from build123d import *

# Parameters (mm, degrees)
CUT_EXTRUDE1_DEPTH = 2.5
FILLET1_R          = 0.5
CHAMFER1_SIZE      = 0.5


with BuildPart() as part:
    # Sketch1 → Revolve1 (revolve)
    with BuildSketch(Plane.XY, mode=Mode.PRIVATE) as revolve1_sk:
        Polygon((0, 0), (-6, 0), (-6, -0.5), (-3, -3.397066324), (-3, -12), (0, -12), align=None)
    revolve(revolve1_sk.sketch.rotate(Axis((0, 0, 0), (0, 1, 0)), 270), axis=Axis((0, 0, 0), (0, 1, 0)))

    # Sketch2 → Cut-Extrude1 (cut)
    with BuildSketch(Plane(origin=(0, 0, 0), x_dir=(1, 0, 0), z_dir=(0, 1, 0))):
        Polygon((0, 2.309401077), (-2, 1.154700538), (-2, -1.154700538), (0, -2.309401077), (2, -1.154700538), (2, 1.154700538), align=None)
    extrude(amount=-CUT_EXTRUDE1_DEPTH, mode=Mode.SUBTRACT)

    # Sketch3 → Cut-Revolve1 (revolve, cut)
    with BuildSketch(Plane.XY, mode=Mode.PRIVATE) as cut_revolve1_sk:
        Polygon((-2.31, 0), (-2, -0.260120886), (-2, -2.5), (0, -3.227940469), (0, 0), align=None)
    revolve(cut_revolve1_sk.sketch.rotate(Axis((0, -3.227940469, 0), (0, -1, 0)), 270), axis=Axis((0, -3.227940469, 0), (0, -1, 0)), mode=Mode.SUBTRACT)

    # Fillet1
    fillet1_edges = [part.edges().sort_by_distance(p)[0] for p in [
        (0, -3.397066324, 3),
    ]]
    fillet(fillet1_edges, radius=FILLET1_R)

    # Chamfer1
    chamfer1_edges = [part.edges().sort_by_distance(p)[0] for p in [
        (0, -12, 3),
    ]]
    chamfer(chamfer1_edges, length=CHAMFER1_SIZE)


solid = part.part
Input: part model. Units: mm. Frame: model coordinates. A direction names the side the tool comes from. Round coordinates to 2 decimals unless told otherwise and drop trailing zeros. Order: outer loops, then holes, each group sorted by start corner. A loop starts at its lowest first (then second) coordinate and runs counter-clockwise, first axis right, second up. Notation, with made-up numbers: (-11, 28.5) - (47, 28.5) arc R20 cw to (47, 44.5) - close; hole circle Ø6 at (-31.75, 8.5). An arc over 180 degrees is marked (long way). Answer as a JSON object with one key per item and string values. Group by question number.
(1) Cut plane B-B (y = -4.5). Return loops of the section in (x, z), then the cut area to 3 significant figures.
(2) Material intervals for probe 1 along X at (y, z) = (-4.5, 0); probe 2 along Z at (x, y) = (-1.5, -0.25); probe 3 along Y at (x, z) = (2.25, -3.5), sorted ascending. Write a range as from..to.
(3) Cut plane A-A (y = -2). Return loops of the section in (x, z), then the cut area to 3 significant figures.
(4) Pin query (flat end, axial travel): P1, Ø1, axis at y = -8.5, z = 0, coming from the -X side; P2, Ø0.7, axis at y = -1, z = 0.5, coming from the -X side; P3, Ø1.5, axis at y = -8.5, z = -2.5, coming from the -X side. Return the tip coordinate at first contact, or that it passes through.
(5) Reachability of faces 1 (the face through (2, -1, 0)), 2 (the face through (0, 0, 3)), 3 (the face through (-3, -8, 0)) from +Z, -Z, +X, -X, +Y, -Y: full face, straight path, thin tool, end or side. Return the list, or none.
(6) Draft query along Z for faces 4 (the face through (0, -12, 0)), 5 (the face through (-0.99, -1.23, -1.74)), 6 (the face through (-1.802, -0.254, -5.723)). Return one class per face: released by +Z, released by -Z, zero draft, split by the parting line, or undercut.
Here are the results:
{
 "1": {"outline": "circle Ø6 at (0, 0)", "area": "28.3 mm^2"},
 "2": {"probe 1": "x = -3..3", "probe 2": "z = -5.81..-1.44, 1.44..5.81", "probe 3": "y = -2.28..0"},
 "3": {"outline": "circle Ø8.89 at (0, 0); hole (-2, -1.15) - (0, -2.31) - (2, -1.15) - (2, 1.15) - (0, 2.31) - (-2, 1.15) - close", "area": "48.3 mm^2"},
 "4": {"P1": "stops at x = -3", "P2": "stops at x = -5.82", "P3": "stops at x = -2.44"},
 "5": {"face 1": "+Y", "face 2": "+Z, -Z, +X, -X, +Y", "face 3": "-Y"},
 "6": {"face 4": "zero draft", "face 5": "undercut", "face 6": "split by the parting line"}
}
